Part model, mm, in its own coordinate system. A direction names the side the tool comes from. Give positions to 0.01 mm unless a question says otherwise; leave off trailing zeros. Order: outer loops, then holes, each group sorted by start corner. A loop starts at its lowest first (then second) coordinate and runs counter-clockwise, first axis right, second up. Notation, with made-up numbers: (21, -15) - (33, -15) arc R19 cw to (33, 8) - close; hole circle Ø7 at (3, 57). An arc over 180 degrees is marked (long way). Use one line per item in the form item = value. Start each with the question number.
1. Pin check, flat tips, straight feed: P1, Ø5, axis at y = 11, z = -4.5, coming from the +X side; P2, Ø1.5, axis at y = 2.5, z = -3.5, coming from the -X side; P3, Ø3, axis at x = -7.36, y = 22.87, coming from the +Z side. Stop position of each tip, or through.
2. Band-saw the part on D-D, the plane y = 5.5. List the corners of the cut face in (x, z), plus the area to 3 significant figures.
3. Pull direction Y, two halves, no side cores. Call faces 5 (the face through (-4.011, 12.295, 3.732)), 6 (the face through (0, 0, 0)), 7 (the face through (-5.568, 17.047, -3.768)), 8 (the face through (-9, 29.586, -4)): +Y half, -Y half, draft (parallel to the pull), parting line (faces both ways), or undercut.
4. Band-saw the part on A-A, the plane y = 25.5. List the corners of the cut face in (x, z), plus the area to 3 significant figures.
5. Tool access for faces 1 (the face through (-6.25, 2, 0)), 2 (the face through (-8, 17, -5)), 3 (the face through (0, 5, 0)), 4 (the face through (2.56, 15.48, -3.77)): list every direction of +Z, -Z, +X, -X, +Y, -Y with a clear straight run to the whole face (end or side of a thin tool).
6. Band-saw the part on B-B, the plane x = 1.5. List the corners of the cut face in (y, z), plus the area to 3 significant figures.
7. Drill centre lines: line 1 (Z direction, x = 4.25, y = 6.75); line 2 (X direction, y = 27.75, z = 2.75); line 3 (Y direction, x = -6, z = 4.5). Where is each one in solid material? Low to high.
8. Band-saw the part on C-C, the plane z = -3.5. List the corners of the cut face in (x, y), plus the area to 3 significant figures.
from build123d import *

# Parameters (mm, degrees)
SKETCH1_W           = 12.5
SKETCH1_H           = 15
BOSS_EXTRUDE1_DEPTH = 5
SKETCH12_R          = 1.1
BOSS_EXTRUDE3_DEPTH = 10
CUT_EXTRUDE2_REACH  = 38.305
SKETCH13_W          = 40
SKETCH13_H          = 5
FILLET2_R           = 5


with BuildPart() as part:
    # Sketch1 → Boss-Extrude1 (new body)
    with BuildSketch(Plane(origin=(0, 0, 0), x_dir=(1, 0, 0), z_dir=(0, 1, 0))):
        Rectangle(SKETCH1_W, SKETCH1_H)
    extrude(amount=BOSS_EXTRUDE1_DEPTH)

    # Sketch12 → Boss-Extrude3 (add)
    with BuildSketch(Plane(origin=(0, 0, -5), x_dir=(-1, 0, 0), z_dir=(0, 0, -1))):
        with BuildLine():
            Line((19.657908058, 29.586368397), (1.407908058, 29.586368397))
            ThreePointArc((1.407908058, 29.586368397), (-2.024927187, 17.169805211), (-6.25, 5))
            Line((-6.25, 5), (6.25, 5))
            ThreePointArc((6.25, 5), (13.739573521, 16.86475517), (19.657908058, 29.586368397))
        make_face()
        with Locations((4.249543893, 13.369198977)):
            Circle(SKETCH12_R, mode=Mode.SUBTRACT)
        with Locations((5.806784348, 18.120514812)):
            Circle(SKETCH12_R, mode=Mode.SUBTRACT)
        with Locations((7.364024803, 22.871830647)):
            Circle(SKETCH12_R, mode=Mode.SUBTRACT)
        with Locations((8.921265258, 27.623146482)):
            Circle(SKETCH12_R, mode=Mode.SUBTRACT)
    extrude(amount=-BOSS_EXTRUDE3_DEPTH)

    # Cut-Extrude2: up to this face of the body (flat: up to its plane)
    cut_extrude2_end = Plane(part.part.faces().sort_by_distance((0, 5, 6.25))[0])
    # Sketch13 → Cut-Extrude2 (cut, up to the picked face)
    with BuildSketch(Plane(origin=(0, 29.586368397, 0), x_dir=(1, 0, 0), z_dir=(0, 1, 0)), mode=Mode.PRIVATE) as cut_extrude2_sk1:
        Rectangle(SKETCH13_W, SKETCH13_H)
    cut_extrude2_tool1 = split(extrude(cut_extrude2_sk1.sketch, amount=-CUT_EXTRUDE2_REACH, mode=Mode.PRIVATE), bisect_by=cut_extrude2_end, keep=Keep.BOTH, mode=Mode.PRIVATE)
    add(cut_extrude2_tool1.solids().sort_by(Axis((0, 29.586368, 0), (0, -1, 0)))[0], mode=Mode.SUBTRACT)

    # Fillet2
    # the kernel refuses this fillet: 5 mm, written as the material it takes off along each edge
    with BuildSketch(Plane(origin=(-19.657908058, 29.586368397, -16.938005308), x_dir=(0.3958255754909857, -0.9183257122542251, 0), z_dir=(0, 0, 1)), Plane(origin=(-19.657908058, 29.586368397, -24.438005308), x_dir=(0.3958255754909857, -0.9183257122542251, 0), z_dir=(0, 0, 1))) as fillet2_piece_1:
        with BuildLine():
            CenterArc((7.598492984, 4.996876412), FILLET2_R, 156.682526959, 115.342832392)
            Line((3.006864423, 6.97600429), (2.915031851, 7.015586847))
            Line((2.915031851, 7.015586847), (-0.091832571, 0.039582558))
            Line((-0.091832571, 0.039582558), (-0.003534183, -0.099937528))
            ThreePointArc((-0.003534183, -0.099937528), (3.887601062, -0.168718929), (7.778736306, -0.099937528))
            Line((7.778736306, -0.099937528), (7.775202123, 0))
        make_face()
    extrude(amount=41.376010616, mode=Mode.SUBTRACT)
    with BuildSketch(Plane(origin=(-1.407908058, 29.586368397, -7.237373954), x_dir=(0.2446328232402741, -0.96961579081278, 0), z_dir=(0, 0, 1)), Plane(origin=(-1.407908058, 29.586368397, -14.737373954), x_dir=(0.2446328232402737, -0.9696157908127802, 0), z_dir=(0, 0, 1))) as fillet2_piece_2:
        with BuildLine():
            CenterArc((3.895246442, -4.999768735), FILLET2_R, 90.551073141, 75.28879109)
            Line((-0.952832513, -3.776604619), (-1.049794092, -3.752141336))
            Line((-1.049794092, -3.752141336), (-0.096961579, 0.024463282))
            Line((-0.096961579, 0.024463282), (0.000961789, 0.099995375))
            ThreePointArc((0.000961789, 0.099995375), (1.92357849, 0.090749401), (3.84619519, 0.099995375))
            Line((3.84619519, 0.099995375), (3.847156979, 0))
        make_face()
    extrude(amount=21.974747908, mode=Mode.SUBTRACT)
    with BuildSketch(Plane(origin=(17.075317547, 5, -7.5), x_dir=(0, -1, 0), z_dir=(-1, 0, 0)), Plane(origin=(-17.075317547, 5, 7.5), x_dir=(0, -1, 0), z_dir=(1, 0, 0))) as fillet2_piece_3:
        with BuildLine():
            CenterArc((4.330127019, 5), FILLET2_R, 210, 60)
            Line((0, 2.5), (-0.08660254, 2.45))
            ThreePointArc((-0.08660254, 2.45), (-0.1, 1.25), (-0.1, 0))
            Line((-0.1, 0), (0, -0.1))
            Line((0, -0.1), (4.330127019, -0.1))
            Line((4.330127019, -0.1), (4.330127019, 0))
        make_face()
    extrude(amount=34.150635095, mode=Mode.SUBTRACT)


solid = part.part
From the geometry:
q1.P1 = 4.94
q1.P2 = -6.25
q1.P3 = 5
q2.outline = (-6.61, -5) - (6.06, -5) - (6.06, -2.5) - (-6.61, -2.5) - close; (-6.61, 2.5) - (6.06, 2.5) - (6.06, 5) - (-6.61, 5) - close
q2.area = 63.3 mm²
q3.face_5 = undercut
q3.face_6 = -Y half
q3.face_7 = undercut
q3.face_8 = +Y half
q4.outline = (-16.98, -5) - (-0.37, -5) - (-0.37, -2.5) - (-16.98, -2.5) - close; (-16.98, 2.5) - (-0.37, 2.5) - (-0.37, 5) - (-16.98, 5) - close
q4.area = 83.0 mm²
q5.face_1 = +Z, -Z, -X, -Y
q5.face_2 = -Z, +X, -X, +Y
q5.face_3 = +X, -X, +Y
q5.face_4 = +Z, -Z, +X, +Y
q6.outline = (0, -7.5) - (0.67, -7.5) arc R5 ccw to (5, -5) - (18.88, -5) - (18.88, -2.5) - (5, -2.5) - (5, 2.5) - (18.88, 2.5) - (18.88, 5) - (5, 5) arc R5 ccw to (0.67, 7.5) - (0, 7.5) - close
q6.area = 138 mm²
q7.line_1 = -5 to -2.5, 2.5 to 5
q7.line_2 = -15.93 to -10.01, -7.83 to -1.43
q7.line_3 = 0 to 17.04, 19.2 to 29.59
q8.outline = (-16.58, 22.45) arc R110 ccw to (-6.25, 5) - (-6.25, 0) - (6.25, 0) - (6.25, 5) arc R200 cw to (-0.47, 25.86) arc R5 ccw to (-5.3, 29.59) - (-12.06, 29.59) arc R5 ccw to start; hole circle Ø2.2 at (-8.92, 27.62); hole circle Ø2.2 at (-7.36, 22.87); hole circle Ø2.2 at (-5.81, 18.12); hole circle Ø2.2 at (-4.25, 13.37)
q8.area = 418 mm²
